CAD build for the part. Positions are in the model's coordinates, mm. A direction names the side the tool comes from. Coordinates: 2 decimals unless noted, no trailing zeros. Write each loop counter-clockwise with the first axis right and the second up, starting at its lowest first coordinate (ties: lowest second). Pieces come first, ordered by that corner, then holes. Notation, with made-up numbers: (-16.5, 68.5) - (-4.5, 68.5) arc R26 cw to (-4.5, 97.5) - close; hole circle Ø3 at (76.5, 84.5). An arc over 180 degrees is marked (long way). Answer in a Markdown table with one row per item. Add a question column.
Q1. Band-saw the part on C-C (x = -1). List the corners of the cut face in (y, z).
Q2. Band-saw the part on B-B (z = 24.5). List the corners of the cut face in (x, y), and give its area (3 significant figures).
Q3. 3-axis set-ups, long thin cutter, end or side, ignore diameter. For faces 5 (the flat face through (-1, 12, -38.1)), 6 (the flat face through (-1, 38.1, 7)): which of +Z, -Z, +X, -X, +Y, -Y reach the whole face in a straight line?
Q4. Drill centre lines: line 1 along X through (y, z) = (-13, -15); line 2 along Y through (x, z) = (28.5, 10); line 3 along Z through (x, y) = (-25.5, 3). Where is each one in solid material? Low to high. Write a range as from..to.
Q5. Two-plate mould, pull along X, no slides. Class faces 1 (the flat face through (7, 41, 38.1)), 2 (the flat face through (-38.1, 6, 6)), 3 (the flat face through (38.1, 6, 6)), 4 (the flat face through (50.8, 12, -1)): +X half, -X half, draft (parallel to the pull), parting line (faces both ways), or undercut.
Q6. Band-saw the part on A-A (y = 33.5). List the corners of the cut face in (x, z), and give its area (3 significant figures).
Q7. Pin check, flat tips, straight feed: pin 1 (5 mm diameter, centred on x = -17.5, z = 13.5, fed in from -Y); pin 2 (4 mm diameter, centred on x = 7, y = 10.5, fed in from +Z). Stop position of each tip, or through.
```python
from build123d import *

# Parameters (mm, degrees)
F0_W          = 101.6
F0_H          = 76.2
F1_DEPTH      = 50.8
F1_DEPTH_BACK = 50.8
F2_T          = -12.7
F1_FACE_W     = 101.6
F1_FACE_H     = 76.2
F3_DEPTH      = 25.4


with BuildPart() as f1:
    # F0 (on Front) → F1 (new body, two sides)
    with BuildSketch(Plane.XZ) as f1_sk:
        Rectangle(F0_W, F0_H)
    extrude(amount=F1_DEPTH)
    extrude(f1_sk.sketch, amount=-F1_DEPTH_BACK)

    # F2
    f2_openings = [f1.faces().sort_by_distance(p)[0] for p in [
        (0, 0, 38.1),
    ]]
    offset(amount=F2_T, openings=f2_openings)

    # F1_face (on face) → F3 (cut)
    with BuildSketch(Plane.XZ.offset(50.8)):
        Rectangle(F1_FACE_W, F1_FACE_H)
    extrude(amount=-F3_DEPTH, mode=Mode.SUBTRACT)


solid = f1.part
```
Checked values:
| question | item | result |
|---|---|---|
| 1 | outline | (-25.4, -38.1) - (50.8, -38.1) - (50.8, 38.1) - (38.1, 38.1) - (38.1, -25.4) - (-25.4, -25.4) - close |
| 2 | outline | (-50.8, -25.4) - (-38.1, -25.4) - (-38.1, 38.1) - (38.1, 38.1) - (38.1, -25.4) - (50.8, -25.4) - (50.8, 50.8) - (-50.8, 50.8) - close |
| 2 | area | 2,900 mm² |
| 3 | face 5 | -Z, +X, -X, +Y, -Y |
| 3 | face 6 | +Z, -Y |
| 4 | line 1 | x = -50.8..-38.1, 38.1..50.8 |
| 4 | line 2 | y = 38.1..50.8 |
| 4 | line 3 | z = -38.1..-25.4 |
| 5 | face 1 | draft |
| 5 | face 2 | undercut |
| 5 | face 3 | undercut |
| 5 | face 4 | +X half |
| 6 | outline | (-50.8, -38.1) - (50.8, -38.1) - (50.8, 38.1) - (38.1, 38.1) - (38.1, -25.4) - (-38.1, -25.4) - (-38.1, 38.1) - (-50.8, 38.1) - close |
| 6 | area | 2,900 mm² |
| 7 | pin 1 | stops at y = 38.1 |
| 7 | pin 2 | stops at z = -25.4 |
